from build123d import *

# Parameters (mm, degrees)
EXTRUDE1_DEPTH      = 56
SKETCH2_R           = 2.5
EXTRUDE2_DEPTH      = 69.585712798
SKETCH4_R           = 10
EXTRUDE3_DEPTH      = 51
FILLET1_R           = 3
SKETCH5_R           = 19
EXTRUDE4_DEPTH      = 1.6
SKETCH6_R           = 3.175
EXTRUDE5_DEPTH      = 20.6
FILLET2_R           = 0.5
SKETCH_1_W          = 0.754278007
SKETCH_1_H          = 3.431599036
CUT_EXTRUDE_1_DEPTH = 2.5


with BuildPart() as part:
    # Sketch1 → Extrude1 (new body)
    with BuildSketch(Plane(origin=(0, 0, 0), x_dir=(1, 0, 0), z_dir=(0, 1, 0))):
        with BuildLine():
            Line((-23, 28), (23, 28))
            ThreePointArc((23, 28), (26.535533906, 26.535533906), (28, 23))
            Line((28, 23), (28, -23))
            ThreePointArc((28, -23), (26.535533906, -26.535533906), (23, -28))
            Line((23, -28), (-23, -28))
            ThreePointArc((-23, -28), (-26.535533906, -26.535533906), (-28, -23))
            Line((-28, -23), (-28, 23))
            ThreePointArc((-28, 23), (-26.535533906, 26.535533906), (-23, 28))
        make_face()
    extrude(amount=EXTRUDE1_DEPTH)

    # Sketch2 → Extrude2 (cut, through all)
    with BuildSketch(Plane.XZ):
        with Locations(Location((23.57, 23.57, 0), (0, 0, 90))):
            Circle(SKETCH2_R)
        with Locations(Location((23.57, -23.57, 0), (0, 0, 270))):
            Circle(SKETCH2_R)
        with Locations(Location((-23.57, -23.57, 0), (0, 0, 90))):
            Circle(SKETCH2_R)
        with Locations(Location((-23.57, 23.57, 0), (0, 0, 270))):
            Circle(SKETCH2_R)
    extrude(amount=-EXTRUDE2_DEPTH, mode=Mode.SUBTRACT)

    # Sketch4 → Extrude3 (cut)
    with BuildSketch(Plane.XZ):
        with Locations((-26.535533906, 26.535533906)):
            Circle(SKETCH4_R)
        with Locations((26.535533906, 26.535533906)):
            Circle(SKETCH4_R)
        with Locations((26.535533906, -26.535533906)):
            Circle(SKETCH4_R)
        with Locations((-26.535533906, -26.535533906)):
            Circle(SKETCH4_R)
    extrude(amount=-EXTRUDE3_DEPTH, mode=Mode.SUBTRACT)

    # Fillet1
    fillet1_edges = [part.edges().sort_by_distance(p)[0] for p in [
        (-28, 25.5, 16.643348149),
        (-16.643348149, 25.5, 28),
        (16.643348149, 25.5, 28),
        (28, 25.5, 16.643348149),
        (28, 25.5, -16.643348149),
        (16.643348149, 25.5, -28),
        (-28, 25.5, -16.643348149),
        (-16.643348149, 25.5, -28),
    ]]
    fillet(fillet1_edges, radius=FILLET1_R)

    # Sketch5 → Extrude4 (add)
    with BuildSketch(Plane(origin=(0, 56, 0), x_dir=(1, 0, 0), z_dir=(0, 1, 0))):
        with Locations(Location((0, 0, 0), (0, 0, 90))):
            Circle(SKETCH5_R)
    extrude(amount=EXTRUDE4_DEPTH)

    # Sketch6 → Extrude5 (add)
    with BuildSketch(Plane(origin=(0, 56, 0), x_dir=(1, 0, 0), z_dir=(0, 1, 0))):
        with Locations(Location((0, 0, 0), (0, 0, 90))):
            Circle(SKETCH6_R)
    extrude(amount=EXTRUDE5_DEPTH)

    # Fillet2
    fillet2_edges = [part.edges().sort_by_distance(p)[0] for p in [
        (0, 76.6, 3.175),
    ]]
    fillet(fillet2_edges, radius=FILLET2_R)

    # Эскиз1 → Вытянуть1 (cut)
    with BuildSketch(Plane(origin=(0, 70.4, 0), x_dir=(-1, 0, 0), z_dir=(0, 1, 0))):
        with Locations((3.096320075, 0.076690216)):
            Rectangle(SKETCH_1_W, SKETCH_1_H)
        with Locations((-3.096320075, 0.076690216)):
            Rectangle(SKETCH_1_W, SKETCH_1_H)
    extrude(amount=CUT_EXTRUDE_1_DEPTH, mode=Mode.SUBTRACT)


solid = part.part
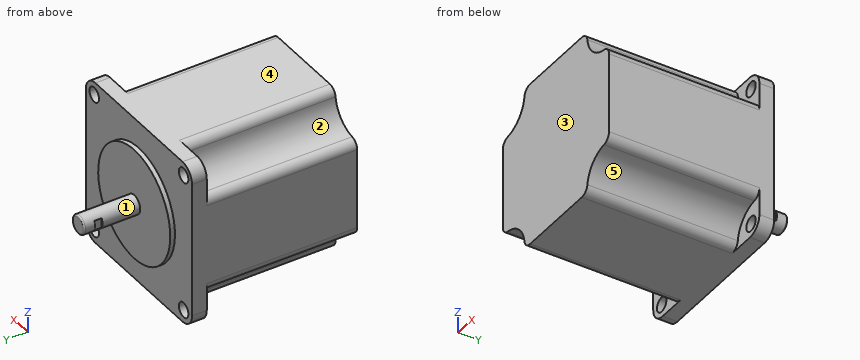
Work out the finished part from the listing and answer in its coordinate system (mm). Face numbers are marked on the shaded views. A direction names the side the tool comes from. Coordinates: 2 decimals unless noted, no trailing zeros. Order: outer loops, then holes, each group sorted by start corner. A loop starts at its lowest first (then second) coordinate and runs counter-clockwise, first axis right, second up. Notation, with made-up numbers: (-9, -1.5) - (22, -1.5) arc R19 ccw to (22, 14.5) - close; hole circle Ø2 at (86.5, 22). An arc over 180 degrees is marked (long way). Put each result on its own line as item: value. Start each with the question number.
1) Find section A-A (x = -22). Give the vertices of the cut face in (y, z).
2) For the marked faces 1, 2, 3, 4 and 5, determine the directions among +Z, -Z, +X, -X, +Y, -Y from which every point of the face is accessible in a straight line to the end or side of a thin tool.
3) Find section C-C (y = 43.5). Give the vertices of the cut face in (x, z), plus the area to 3 significant figures.
4) Find section B-B (z = 0). Give the vertices of the cut face in (x, y) (3 decimals), plus the area to 3 significant figures.
5) Flat-ended cylindrical pins translate along their axes: pin 1 (4 mm diameter, centred on y = 14.5, z = 16.5, fed in from +X); pin 2 (6 mm diameter, centred on x = -23.57, z = -23.57, fed in from +Y); pin 3 (4 mm diameter, centred on x = 23.57, z = -23.57, fed in from +Y); pin 4 (2 mm diameter, centred on y = 44, z = 14, fed in from +X). Find the tip coordinate at first contact, or state that the pin passes through.
6) Find the intervals of material crossed by line 1 (X direction, y = 54.6, z = -23.57); line 2 (Z direction, x = -23, y = 54), in increasing order. Write a range as from..to.
7) Find section D-D (x = 9). Give the vertices of the cut face in (y, z), plus the area to 3 significant figures.
Results list:
1. outline: (0, -17.62) - (51, -17.62) - (51, -21.62) - (56, -21.62) - (56, 21.62) - (51, 21.62) - (51, 17.62) - (0, 17.62) - close; (51, -28) - (56, -28) - (56, -25.52) - (51, -25.52) - close; (51, 25.52) - (56, 25.52) - (56, 28) - (51, 28) - close
2. face 1: +Y
2. face 2: +Z, -X, -Y
2. face 3: +Z, -Z, +X, -X, -Y
2. face 4: +Z, +X, -X, +Y, -Y
2. face 5: -Z, +X, -Y
3. outline: (-28, -13.63) arc R3 ccw to (-25.35, -16.61) arc R10 cw to (-16.61, -25.35) arc R3 ccw to (-13.63, -28) - (13.63, -28) arc R3 ccw to (16.61, -25.35) arc R10 cw to (25.35, -16.61) arc R3 ccw to (28, -13.63) - (28, 13.63) arc R3 ccw to (25.35, 16.61) arc R10 cw to (16.61, 25.35) arc R3 ccw to (13.63, 28) - (-13.63, 28) arc R3 ccw to (-16.61, 25.35) arc R10 cw to (-25.35, 16.61) arc R3 ccw to (-28, 13.63) - close
3. area: 2,680 mm^2
4. outline: (-28, 0) - (28, 0) - (28, 56) - (19, 56) - (19, 57.6) - (3.175, 57.6) - (3.175, 70.4) - (2.719, 70.4) - (2.719, 72.9) - (3.175, 72.9) - (3.175, 76.1) arc R0.5 ccw to (2.675, 76.6) - (-2.675, 76.6) arc R0.5 ccw to (-3.175, 76.1) - (-3.175, 72.9) - (-2.719, 72.9) - (-2.719, 70.4) - (-3.175, 70.4) - (-3.175, 57.6) - (-19, 57.6) - (-19, 56) - (-28, 56) - close
4. area: 3,320 mm^2
5. pin 1: stops at x = 27.87
5. pin 2: stops at y = 56
5. pin 3: passes through
5. pin 4: stops at x = 28
6. line 1: x = -27.97..-26.07, -21.07..21.07, 26.07..27.97
6. line 2: z = -28..-26, -21.14..21.14, 26..28
7. outline: (0, -28) - (56, -28) - (56, -16.73) - (57.6, -16.73) - (57.6, 16.73) - (56, 16.73) - (56, 28) - (0, 28) - close
7. area: 3,190 mm^2
